Check sheet for the modelled part. Datum: model origin and axes. Units: mm. Face numbers are marked on the shaded views. A direction names the side the tool comes from. Coordinates: 2 decimals unless noted, no trailing zeros. Loops run counter-clockwise (first coordinate to the right, second up) from the corner with the lowest first, then second, coordinate; pieces in that order, holes last.
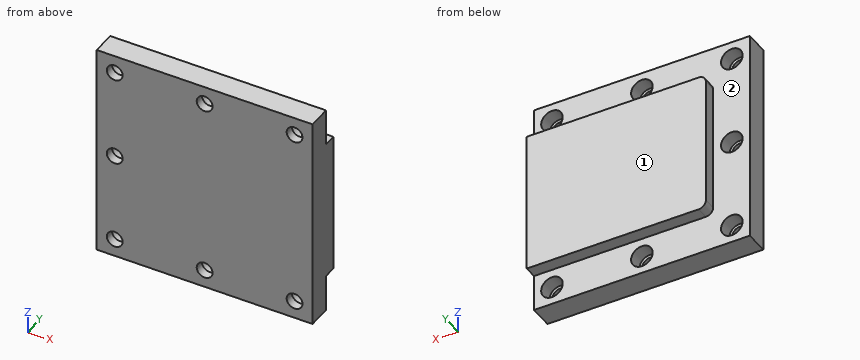
Autodesk Inventor part; units mm, degrees
ref_plane "YZ Plane" through (0, 0, 0) normal (1, 0, 0) x (0, 1, 0)
ref_plane "XZ Plane" through (0, 0, 0) normal (0, 1, 0) x (-1, 0, 0)
ref_plane "XY Plane" through (0, 0, 0) normal (0, 0, 1) x (1, 0, 0)
sketch "Sketch1" plane through (0, 0, 0) normal (0, 1, 0) x (-1, 0, 0)
  line L0 (-15, -15) -> (15, -15)
  line L1 (15, -15) -> (15, 15)
  line L2 (15, 15) -> (-15, 15)
  line L3 (-15, 15) -> (-15, -15)
  line L4 (-15, -15) -> (15, 15) construction
  line L5 (15, -15) -> (-15, 15) construction
  point P0 (0, 0)
  dimension "d0" = 30
  dimension "d1" = 30
extrude "Extrusion1" add sketch "Sketch1" along normal blind 5
sketch "Sketch2" plane through (0, 5, 0) normal (0, 1, 0) x (1, 0, 0)
  line L0 (-15, -15) -> (15, -15)
  line L1 (-15, 15) -> (-15, -15)
  line L2 (15, 15) -> (-15, 15)
  line L3 (15, -15) -> (15, 15)
  line L4 (-15, -15) -> (15, -15)
  line L5 (15, -15) -> (15, -9.9)
  line L6 (15, -9.9) -> (-8.9, -9.9)
  line L7 (-15, -9.9) -> (-15, -15)
  line L8 (-15, -15) -> (-9.9, -15)
  line L9 (-9.9, -8.9) -> (-9.9, 8.9)
  line L10 (-9.9, 15) -> (-15, 15)
  line L11 (-15, 15) -> (-15, -15)
  line L12 (15, 15) -> (-9.9, 15)
  line L13 (-9.9, 15) -> (-9.9, 9.9)
  line L14 (-8.9, 9.9) -> (15, 9.9)
  line L15 (15, 9.9) -> (15, 15)
  arc A0 (-9.9, -8.9) -> (-8.9, -9.9) centre (-8.9, -8.9) ccw
  arc A1 (-8.9, 9.9) -> (-9.9, 8.9) centre (-8.9, 8.9) ccw
  point P0 (0, 0)
  dimension "d4" = 5.1
  dimension "d5" = 5.1
  dimension "d6" = 5.1
  dimension "d7" = 1
extrude "Extrusion2" cut sketch "Sketch2" against normal blind 1.75 contours L1 L2 L3 L14 A1 L9 A0 L6 L0
sketch "Sketch3" plane through (0, 3.25, 0) normal (0, 1, 0) x (1, 0, 0)
  line L0 (-9.9, 8.9) -> (-9.9, -8.9)
  line L1 (15, -15) -> (-15, -15)
  line L2 (-15, 15) -> (15, 15)
  point P0 (0, 0)
  point P1 (-12.5, -12.5)
  point P2 (12.5, -12.5)
  point P3 (-12.5, 12.5)
  point P4 (12.5, 12.5)
  point P5 (-9.9, 0)
  point P6 (0, -15)
  point P7 (0, -12.5)
  point P8 (-12.5, 0)
  point P9 (0, 12.5)
  point P10 (-9.9, 0)
  point P11 (0, -15)
  point P12 (0, 15)
  dimension "d10" = 25
  dimension "d11" = 25
  dimension "d12" = 12.5
  dimension "d13" = 12.5
hole "Hole1" at (-12.5, 3.25, 12.5) at (12.5, 3.25, 12.5) at (-12.5, 3.25, -12.5) at (12.5, 3.25, -12.5) at (0, 3.25, 12.5) at (0, 3.25, -12.5) at (-12.5, 3.25, 0) direction (0, -1, 0) diameter 3 depth 2
hole "Hole2" at (-12.5, 3.25, 0) at (-12.5, 3.25, 12.5) at (0, 3.25, 12.5) at (12.5, 3.25, 12.5) at (12.5, 3.25, -12.5) at (0, 3.25, -12.5) at (-12.5, 3.25, -12.5) direction (0, -1, 0) diameter 2.2 end through all
equation "\"d5\" = d4"
equation "\"d6\" = d4"
properties part number "Flex Circuit Clamp Base V1"
(1) Gauge pin test, flat ends, axial feed: P1, Ø1.8, axis at x = -12.5, z = -12.5, coming from the +Y side; P2, Ø0.5, axis at x = 5.5, y = 4, coming from the -Z side; P3, Ø5, axis at x = -12.5, z = 0, coming from the +Y side; P4, Ø2.5, axis at x = 12.5, z = 12.5, coming from the +Y side. Record the tip position at first contact, or that the pin passes through.
(2) Section check C-C, the plane x = -12.5. Enter the section's corners in (y, z), plus the area to 4 significant figures.
(3) Section check A-A, the plane z = -12.5. Enter the section's corners in (x, y), plus the area to 4 significant figures.
(4) Section check D-D, the plane x = 0. Enter the section's corners in (y, z), plus the area to 3 significant figures.
(5) Scan lines: line 1 along Z through (x, y) = (12.5, 0.4); line 2 along Z through (x, y) = (-12.5, 2.85). Record each from-to range of solid material in increasing order.
(6) Set-up check for the marked faces 1 and 2: record each of +Z, -Z, +X, -X, +Y, -Y from which the full face is reachable in a straight line by a thin tool's end or side.
(7) Section check B-B, the plane y = 2.2. Enter the section's corners in (x, z), plus the area to 3 significant figures.
Determined:
1. P1: passes through
1. P2: stops at z = -9.9
1. P3: stops at y = 3.25
1. P4: stops at y = 1.25
2. outline: (0, -15) - (3.25, -15) - (3.25, -14) - (1.25, -14) - (1.25, -13.6) - (0, -13.6) - close; (0, -11.4) - (1.25, -11.4) - (1.25, -11) - (3.25, -11) - (3.25, -1.5) - (1.25, -1.5) - (1.25, -1.1) - (0, -1.1) - close; (0, 1.1) - (1.25, 1.1) - (1.25, 1.5) - (3.25, 1.5) - (3.25, 11) - (1.25, 11) - (1.25, 11.4) - (0, 11.4) - close; (0, 13.6) - (1.25, 13.6) - (1.25, 14) - (3.25, 14) - (3.25, 15) - (0, 15) - close
2. area: 71.25 mm2
3. outline: (-15, 0) - (-13.6, 0) - (-13.6, 1.25) - (-14, 1.25) - (-14, 3.25) - (-15, 3.25) - close; (-11.4, 0) - (-1.1, 0) - (-1.1, 1.25) - (-1.5, 1.25) - (-1.5, 3.25) - (-11, 3.25) - (-11, 1.25) - (-11.4, 1.25) - close; (1.1, 0) - (11.4, 0) - (11.4, 1.25) - (11, 1.25) - (11, 3.25) - (1.5, 3.25) - (1.5, 1.25) - (1.1, 1.25) - close; (13.6, 0) - (15, 0) - (15, 3.25) - (14, 3.25) - (14, 1.25) - (13.6, 1.25) - close
3. area: 71.25 mm2
4. outline: (0, -15) - (3.25, -15) - (3.25, -14) - (1.25, -14) - (1.25, -13.6) - (0, -13.6) - close; (0, -11.4) - (1.25, -11.4) - (1.25, -11) - (3.25, -11) - (3.25, -9.9) - (5, -9.9) - (5, 9.9) - (3.25, 9.9) - (3.25, 11) - (1.25, 11) - (1.25, 11.4) - (0, 11.4) - close; (0, 13.6) - (1.25, 13.6) - (1.25, 14) - (3.25, 14) - (3.25, 15) - (0, 15) - close
4. area: 115 mm2
5. line 1: z = -15 to -13.6, -11.4 to 11.4, 13.6 to 15
5. line 2: z = -15 to -14, -11 to -1.5, 1.5 to 11, 14 to 15
6. face 1: +Z, -Z, +X, -X, +Y
6. face 2: -X, +Y
7. outline: (-15, -15) - (15, -15) - (15, 15) - (-15, 15) - close; hole circle Ø3 at (-12.5, -12.5); hole circle Ø3 at (-12.5, 0); hole circle Ø3 at (-12.5, 12.5); hole circle Ø3 at (0, -12.5); hole circle Ø3 at (0, 12.5); hole circle Ø3 at (12.5, -12.5); hole circle Ø3 at (12.5, 12.5)
7. area: 851 mm2
